For this review, take the finished solid that the model builds, in its own axes (mm). Coordinates: 2 decimals unless noted, no trailing zeros. Write each loop counter-clockwise with the first axis right and the second up, starting at its lowest first coordinate (ties: lowest second). Pieces come first, ordered by that corner, then holes. Notation, with made-up numbers: (21, 39.5) -> (63, 39.5) arc R22 cw to (63, 56.5) -> close; hole circle Ø6 at (20.5, 6). An arc over 180 degrees is marked (long way). One line per item, written item: value. Start each with the question number.
1) For probe 1 along X at (y, z) = (-3, 2.5); probe 2 along X at (y, z) = (-0.25, 7); probe 3 along Z at (x, y) = (-7, -7.5), list the stretches that pass through material, from the lowest coordinate up. Write a range as from..to.
2) Add section D-D (z = 2.5). State the section outline as (x, y) points.
3) Add section B-B (z = 6.4). State the section outline as (x, y) points.
4) Mouldability with a two-part tool opening along Z and no side actions: class faces 1 (the cylindrical face through (-11.43, -1.07, 12.5)), 2 (the cylindrical face through (-5.097, 0.265, 2.493)), 3 (the cylindrical face through (-8.408, -1.071, 5.462)) as released by +Z, released by -Z, zero draft, split by the parting line, or undercut.
5) Add section C-C (z = 12.25). State the section outline as (x, y) points.
6) Add section A-A (y = -10.5). State the section outline as (x, z) points, and give its area (3 significant figures).
from build123d import *

# Parameters (mm, degrees)
SKETCH1_W          = 26
SKETCH1_H          = 29.8
EXTRUDE1_DEPTH     = 14.3
FILLET1_R          = 6
SKETCH3_R          = 2.45
CUT_EXTRUDE1_DEPTH = 30.8
SKETCH2_R          = 1.95
EXTRUDE2_DEPTH     = 15.3


with BuildPart() as part:
    # Sketch1 → Extrude1 (new body)
    with BuildSketch(Plane.XY):
        with Locations((-0.145304935, -1.279569379)):
            Rectangle(SKETCH1_W, SKETCH1_H)
    extrude(amount=EXTRUDE1_DEPTH)

    # Fillet1
    fillet1_edges = [part.edges().sort_by_distance(p)[0] for p in [
        (12.854695065, -1.279569379, 14.3),
        (-13.145304935, -1.279569379, 14.3),
    ]]
    fillet(fillet1_edges, radius=FILLET1_R)

    # Sketch3 → Cut-Extrude1 (cut, through all)
    with BuildSketch(Plane(origin=(0, 13.620430621, 0), x_dir=(-1, 0, 0), z_dir=(0, 1, 0))):
        with Locations((-7.854695065, 6.4000002)):
            Circle(SKETCH3_R)
        with Locations((6.145304935, 6.4)):
            Circle(SKETCH3_R)
    extrude(amount=-CUT_EXTRUDE1_DEPTH, mode=Mode.SUBTRACT)

    # Sketch2 → Extrude2 (cut, through all)
    with BuildSketch(Plane.XY.offset(14.3)):
        with Locations((-6.145304935, -1.379569379)):
            Circle(SKETCH2_R)
        with Locations((5.854695065, -1.379569379)):
            Circle(SKETCH2_R)
    extrude(amount=-EXTRUDE2_DEPTH, mode=Mode.SUBTRACT)


solid = part.part
Numbers:
1. probe 1: -13.15..-7.23, -5.06..4.77, 6.94..12.85
1. probe 2: -13.15..-8.52, -3.77..4.27, 10.23..12.85
1. probe 3: 0..4.1, 8.7..14.3
2. outline: (-13.15, -16.18) -> (12.85, -16.18) -> (12.85, 13.62) -> (-13.15, 13.62) -> close; hole circle Ø3.9 at (-6.15, -1.38); hole circle Ø3.9 at (5.85, -1.38)
3. outline: (-13.15, -16.18) -> (-8.6, -16.18) -> (-8.6, 13.62) -> (-13.15, 13.62) -> close; (-3.7, -16.18) -> (5.4, -16.18) -> (5.4, -3.28) arc R1.95 cw to (5.4, 0.52) -> (5.4, 13.62) -> (-3.7, 13.62) -> close; (10.3, -16.18) -> (12.85, -16.18) -> (12.85, 13.62) -> (10.3, 13.62) -> close
4. face 1: released by +Z
4. face 2: zero draft
4. face 3: undercut
5. outline: (-11.66, -16.18) -> (11.37, -16.18) -> (11.37, 13.62) -> (-11.66, 13.62) -> close; hole circle Ø3.9 at (-6.15, -1.38); hole circle Ø3.9 at (5.85, -1.38)
6. outline: (-13.15, 0) -> (12.85, 0) -> (12.85, 8.3) arc R6 ccw to (6.85, 14.3) -> (-7.15, 14.3) arc R6 ccw to (-13.15, 8.3) -> close; hole circle Ø4.9 at (-6.15, 6.4); hole circle Ø4.9 at (7.85, 6.4)
6. area: 319 mm²
